Input: dimensioned drawing with shaded views. Units: mm. Origin: part minimum x, y, z. Give positions to 0.01 mm unless a question says otherwise; leave off trailing zeros. Loops run counter-clockwise (first coordinate to the right, second up) from the corner with the lowest first, then second, coordinate; pieces in that order, holes last. Notation, with made-up numbers: M -5,31.5 L 10,31.5 A35 cw 10,65.5 Z; hole C 51.25,4 d3. An arc over 180 degrees is marked long. Answer in a Markdown table with one row per item.
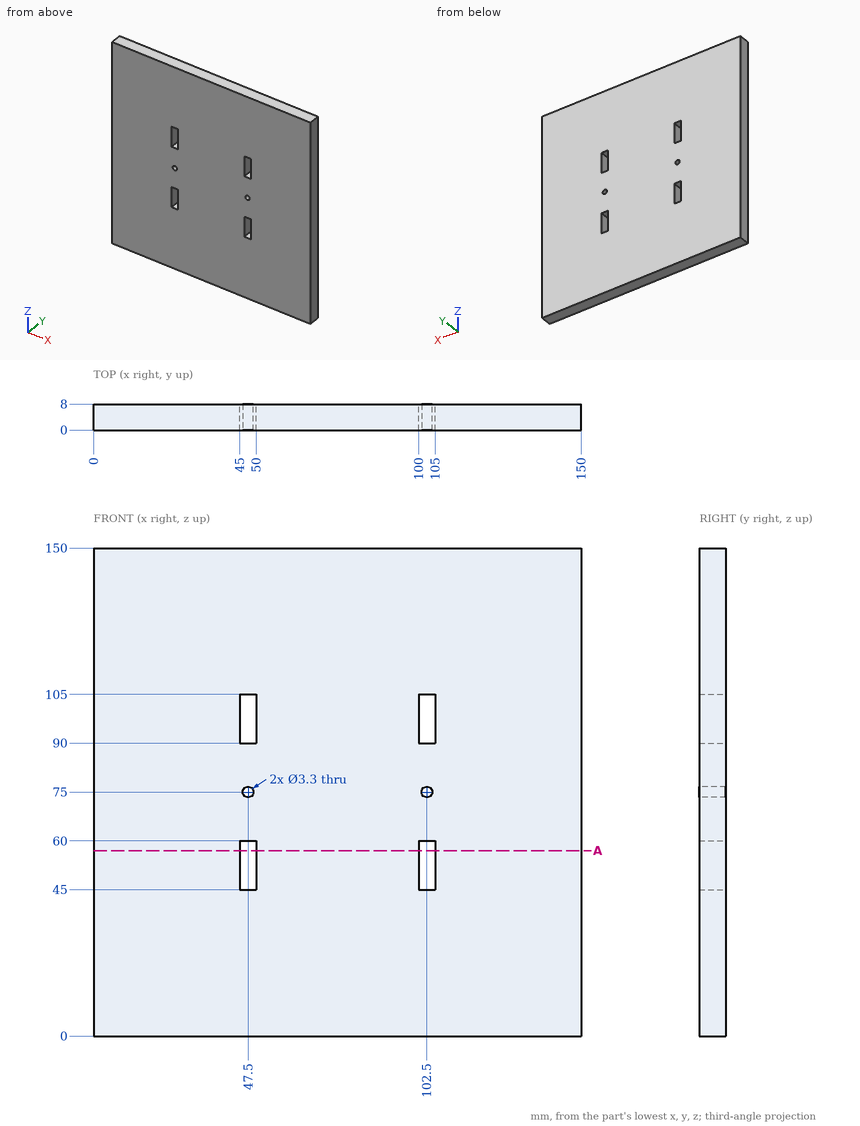
Q1. Section query A-A (z = 57). Output: boundary loops of the cut face in (x, y), plus the area to 3 significant figures.
Values follow:
| item | result |
|---|---|
| outline | M 0,0 L 45,0 L 45,8 L 0,8 Z; M 50,0 L 100,0 L 100,8 L 50,8 Z; M 105,0 L 150,0 L 150,8 L 105,8 Z |
| area | 1,120 mm^2 |
Q2. Contact query for a flat-ended pin moving along its axis: pin 1 Ø4.5 at (x, z) = (47.5, 75) entering from -Y. Output: stop coordinate, or through.
Values follow:
| item | result |
|---|---|
| pin 1 | y = 0 |
Q3. Ray query, probe 1 along X at (y, z) = (3.75, 75); probe 2 along Z at (x, y) = (47.5, 4.25); probe 3 along X at (y, z) = (7.25, 76). Return the intervals inside material, ascending. Write a range as from..to.
Values follow:
| item | result |
|---|---|
| probe 1 | 0..45.85, 49.15..100.85, 104.15..150 |
| probe 2 | 0..45, 60..73.35, 76.65..90, 105..150 |
| probe 3 | 0..46.19, 48.81..101.19, 103.81..150 |
